from build123d import *

# Parameters (mm, degrees)
SKETCH1_W           = 142
SKETCH1_H           = 92
BOSS_EXTRUDE1_DEPTH = 14
FILLET1_R           = 10
SKETCH2_R           = 27.5
SKETCH2_R_2         = 15
BOSS_EXTRUDE2_DEPTH = 22.5
BOSS_EXTRUDE3_DEPTH = 7.5
BOSS_EXTRUDE4_DEPTH = 7.5
SKETCH5_R           = 9
CUT_EXTRUDE1_DEPTH  = 121.279881942


with BuildPart() as part:
    # Sketch1 → Boss-Extrude1 (new body)
    with BuildSketch(Plane(origin=(0, 0, 0), x_dir=(1, 0, 0), z_dir=(0, 1, 0))):
        Rectangle(SKETCH1_W, SKETCH1_H)
    extrude(amount=BOSS_EXTRUDE1_DEPTH)

    # Fillet1
    fillet1_edges = [part.edges().sort_by_distance(p)[0] for p in [
        (-71, 7, -46),
        (71, 7, -46),
        (71, 7, 46),
        (-71, 7, 46),
    ]]
    fillet(fillet1_edges, radius=FILLET1_R)



with BuildPart() as body_2:
    # Sketch2 → Boss-Extrude2 (new, symmetric)
    with BuildSketch(Plane(origin=(0, 0, 0), x_dir=(0, 0, -1), z_dir=(1, 0, 0))):
        with Locations(Location((0, 72, 0), (0, 0, 180))):
            Circle(SKETCH2_R)
        with Locations(Location((0, 72, 0), (0, 0, 180))):
            Circle(SKETCH2_R_2, mode=Mode.SUBTRACT)
    extrude(amount=BOSS_EXTRUDE2_DEPTH, both=True)


with BuildPart() as part_1:
    add(part.part)

    add(body_2.part)  # Boss-Extrude3 merges body 2
    # Sketch3 → Boss-Extrude3 (add, symmetric)
    with BuildSketch(Plane.XY):
        Polygon((0, 49.5), (-22.5, 49.5), (-22.5, 44.5), (-48.5, 14), (-48.5, 6.529967444), (0, 6.529967444), (0, 44.5), align=None)
    extrude(amount=BOSS_EXTRUDE3_DEPTH, both=True)

    # Mirror1: part across plane


with BuildPart() as part_2:
    add(part_1.part)
    add(part_1.part.mirror(Plane(origin=(0, 0, 0), x_dir=(0, 0, 1), z_dir=(1, 0, 0))))

    # Sketch4 → Boss-Extrude4 (add, symmetric)
    with BuildSketch(Plane(origin=(0, 0, 0), x_dir=(0, 0, -1), z_dir=(1, 0, 0))):
        with BuildLine():
            Line((7.5, 14), (36, 14))
            Line((36, 14), (46, 14))
            Line((46, 14), (46, 36))
            Line((46, 36), (27.5, 72))
            ThreePointArc((27.5, 72), (21.937410968, 55.416876048), (7.5, 45.542486889))
            Line((7.5, 45.542486889), (7.5, 44.5))
            Line((7.5, 44.5), (7.5, 14))
        make_face()
    extrude(amount=BOSS_EXTRUDE4_DEPTH, both=True)

    # Mirror3: part across plane


with BuildPart() as part_3:
    add(part_2.part)
    add(part_2.part.mirror(Plane.XY))

    # Sketch5 → Cut-Extrude1 (cut, through all)
    with BuildSketch(Plane(origin=(0, 14, 0), x_dir=(1, 0, 0), z_dir=(0, 1, 0))):
        with Locations(Location((50, -25, 0), (0, 0, 270))):
            Circle(SKETCH5_R)
        with Locations(Location((50, 25, 0), (0, 0, 270))):
            Circle(SKETCH5_R)
        with Locations(Location((-50, 25, 0), (0, 0, 90))):
            Circle(SKETCH5_R)
        with Locations(Location((-50, -25, 0), (0, 0, 90))):
            Circle(SKETCH5_R)
    extrude(amount=-CUT_EXTRUDE1_DEPTH, mode=Mode.SUBTRACT)


solid = part_3.part
Input: part model. Units: mm. Frame: model coordinates. A direction names the side the tool comes from. Coordinates: 2 decimals unless noted, no trailing zeros. Write each loop counter-clockwise with the first axis right and the second up, starting at its lowest first coordinate (ties: lowest second). Pieces come first, ordered by that corner, then holes. Notation, with made-up numbers: M 87.25,34 L 112.25,34 A24 ccw 112.25,46 Z; hole C 25.5,4.25 d10. An arc over 180 degrees is marked long. Answer as a JSON object with one key per item and string values. Group by question number.
(1) Section A-A on z = 0. Output: boundary loops of the cut face in (x, y).
(2) Ray query, line 1 along X through (y, z) = (9.5, 25); line 2 along Z through (x, y) = (-50, 10.25); line 3 along Y through (x, z) = (-14, -11.5). Return the intervals inside material, ascending. Write a range as [from, to].
(3) Set-up query: faces 1 (the face through (7.5, 37, -26)), 2 (the face through (22.5, 84, 12)), 3 (the face through (7.5, 37, 26)). Return all of +Z, -Z, +X, -X, +Y, -Y with unobstructed straight access to the full face (end or side cutting, diameter ignored); none if empty.
(4) Contact query for flat-ended pins moving along their axis: P1, Ø19, axis at y = 37, z = -29.5, coming from the +X side; P2, Ø23.5, axis at x = 50, z = 25, coming from the +Y side; P3, Ø25, axis at x = -30.5, y = 31.5, coming from the -Z side. Output: stop coordinate, or through.
(5) Section B-B on x = -5. Output: boundary loops of the cut face in (y, z), plus the area to 3 significant figures.
(6) Mould query, pull axis Z, two halves, no side actions, for faces 4 (the face through (-57.59, 7.1, -29.84)), 5 (the face through (0.11, 53.75, -36.88)), 6 (the face through (1, 10, 46)). Classes: pulls with the +Z half, pulls with the -Z half, needs draft (parallel to the pull), parting line crosses it, or undercut.
(7) Section D-D on z = -25. Output: boundary loops of the cut face in (x, y), plus the area to 3 significant figures.
(8) Section C-C on y = 69. Output: boundary loops of the cut face in (x, z).
Result set:
{
 "1": {"outline": "M -71,0 L 71,0 L 71,14 L 48.5,14 L 22.5,44.5 L 22.5,57 L -22.5,57 L -22.5,44.5 L -48.5,14 L -71,14 Z; M -22.5,87 L 22.5,87 L 22.5,99.5 L -22.5,99.5 Z"},
 "2": {"line 1": "x = [-71, -59], [-41, 41], [59, 71]", "line 2": "z = [-46, -34], [-16, 16], [34, 46]", "line 3": "y = [0, 14], [47.02, 62.37], [81.63, 96.98]"},
 "3": {"face 1": "-Z, +X", "face 2": "+Z, -Z, +X, +Y", "face 3": "+Z, +X"},
 "4": {"P1": "stops at x = 7.5", "P2": "stops at y = 14", "P3": "stops at z = -7.5"},
 "5": {"outline": "M 0,-46 L 36,-46 L 72,-27.5 A27.5 ccw 72,27.5 L 36,46 L 0,46 Z; hole C 72,0 d30", "area": "6,440 mm2"},
 "6": {"face 4": "undercut", "face 5": "pulls with the -Z half", "face 6": "pulls with the +Z half"},
 "7": {"outline": "M -71,0 L -59,0 L -59,14 L -71,14 Z; M -41,0 L 41,0 L 41,14 L 7.5,14 L 7.5,60.54 L 22.5,60.54 L 22.5,83.46 L -22.5,83.46 L -22.5,60.54 L -7.5,60.54 L -7.5,14 L -41,14 Z; M 59,0 L 71,0 L 71,14 L 59,14 Z", "area": "3,210 mm2"},
 "8": {"outline": "M -22.5,-27.34 L -7.5,-27.34 L -7.5,-29.04 L 7.5,-29.04 L 7.5,-27.34 L 22.5,-27.34 L 22.5,-14.7 L -22.5,-14.7 Z; M -22.5,14.7 L 22.5,14.7 L 22.5,27.34 L 7.5,27.34 L 7.5,29.04 L -7.5,29.04 L -7.5,27.34 L -22.5,27.34 Z"}
}
